Autodesk Fusion 360 part; units mm, degrees
sketch "Sketch1" plane through (0, 0, 0) normal (0, 0, 1) x (1, 0, 0)
  line L0 (44.75, 21) -> (-44.75, 21)
  line L1 (-44.75, 21) -> (-44.75, -21)
  line L2 (-44.75, -21) -> (44.75, -21)
  line L3 (44.75, -21) -> (44.75, 21)
  line L4 (44.75, 21) -> (-44.75, -21) construction
  line L5 (-44.75, 21) -> (44.75, -21) construction
  circle A0 centre (-42.25, 18.5) radius 1.25
  line L6 (20, 0) -> (2.5, 0)
  circle A1 centre (-42.25, -18.5) radius 1.25
  line L7 (0, 2.5) -> (0, 20)
  circle A2 centre (42.25, -18.5) radius 1.25
  circle A3 centre (42.25, 18.5) radius 1.25
  line L8 (38.75, 18.75) -> (-38.75, 18.75)
  line L9 (-38.75, 18.75) -> (-38.75, -18.75)
  line L10 (-38.75, -18.75) -> (38.75, -18.75)
  line L11 (38.75, -18.75) -> (38.75, 18.75)
  line L12 (38.75, 18.75) -> (-38.75, -18.75) construction
  line L13 (-38.75, 18.75) -> (38.75, -18.75) construction
  line L14 (39.75, 19.75) -> (-39.75, 19.75)
  line L15 (-39.75, 19.75) -> (-39.75, -19.75)
  line L16 (-39.75, -19.75) -> (39.75, -19.75)
  line L17 (39.75, -19.75) -> (39.75, 19.75)
  line L18 (39.75, 19.75) -> (-39.75, -19.75) construction
  line L19 (-39.75, 19.75) -> (39.75, -19.75) construction
  line L20 (37.5, 17.5) -> (-37.5, 17.5)
  line L21 (-37.5, 17.5) -> (-37.5, -17.5)
  line L22 (-37.5, -17.5) -> (37.5, -17.5)
  line L23 (37.5, -17.5) -> (37.5, 17.5)
  line L24 (37.5, 17.5) -> (-37.5, -17.5) construction
  line L25 (-37.5, 17.5) -> (37.5, -17.5) construction
  dimension "d5" = 2.5
  dimension "d38" = 75
  dimension "d39" = 35
  dimension "d40" = 3.5
  dimension "d41" = 1.25
  dimension "d42" = 1.25
  dimension "d43" = 1.25
  dimension "d44" = 2.25
  dimension "d45" = 2.5
  dimension "d46" = 2.5
  dimension "d47" = 2.5
extrude "Extrude1" add sketch "Sketch1" along normal blind 2.5 contours L0 L1 L2 L3 | L8 L9 L10 L11 | L14 L15 L16 L17 | L20 L21 L22 L23
extrude "Extrude7" add sketch "Sketch1" along normal blind 5 from surface at 2.5 contours L14 L15 L16 L17
extrude "Extrude8" cut sketch "Sketch1" against normal blind 0.5 from surface at 2.5 contours L20 L21 L22 L23
fillet "Fillet3" radius 2 16 edges at (-39.75, -19.75, 5) (-44.75, -21, 1.25) (-38.75, -18.75, 5) (-37.5, -17.5, 2.25) (-37.5, 17.5, 2.25) (-38.75, 18.75, 5) (-39.75, 19.75, 5) (-44.75, 21, 1.25) (39.75, 19.75, 5) (44.75, 21, 1.25) (39.75, -19.75, 5) (44.75, -21, 1.25) (37.5, -17.5, 2.25) (38.75, -18.75, 5) (38.75, 18.75, 5) (37.5, 17.5, 2.25)
equation "d42 = d41"
equation "d43 = d41"
equation "d44 = d40 - d41"
equation "d45 = d41 + 0.5 * d5"
equation "d46 = d41 + 0.5 * d5"
equation "d47 = d41 + 0.5 * d5"
equation "d48 = d3"
equation "d51 = d3"
Could you check a few things on this model? Use its own coordinates, in mm. A direction names the side the tool comes from. Give positions to 0.01 mm unless a question says otherwise; leave off trailing zeros. Order: outer loops, then holes, each group sorted by start corner. A loop starts at its lowest first (then second) coordinate and runs counter-clockwise, first axis right, second up. Notation, with made-up numbers: (59, 69) - (99, 69) arc R23 cw to (99, 82) - close; hole circle Ø10 at (51.25, 28). An arc over 180 degrees is marked (long way). One line per item, written item: value. Start each with the question number.
1. Imagine slicing it at C-C on y = -13. List the corners of the cut face in (x, z) for me, plus the area to 3 significant figures.
2. Imagine slicing it at B-B on x = -33.5. List the corners of the cut face in (y, z) for me, plus the area to 3 significant figures.
3. Thinking about a two-plate mould opening in X: for faces 1 (the face through (-44.15, 20.43, 1.27)), 2 (the face through (44.18, 20.4, 1.27)), 3 (the face through (-43.24, -17.74, 1.23)), 4 (the face through (0, 19, 7.5)), which applies, +X half, -X half, draft (parallel to the pull), parting line (faces both ways), or undercut?
4. Imagine slicing it at A-A on z = 4.25. List the corners of the cut face in (x, y) for me.
5. If I drill on probe 1 along Y at (x, z) = (-42.25, 1.8); probe 2 along Y at (x, z) = (15, 4); probe 3 along X at (y, z) = (13.5, 3), over which ranges is the centre line in solid material (lowest first)?
6. For P1, Ø1.5, axis at x = -2, z = 5, coming from the -Y side; P2, Ø3, axis at x = -35, y = -14.5, coming from the +Z side; P3, Ø1.5, axis at x = -17, z = 6, coming from the +Y side, each with a flat end and sliding along its axis, tell me the tip position at first contact or that it passes through.
7. For faces 5 (the face through (-39.18, -19.15, 5.04)), 6 (the face through (-1, -19.75, 5)), 7 (the face through (39.75, 0, 5)), 8 (the face through (39.18, 19.15, 5.04)), 9 (the face through (-38.15, 18.18, 5.04)), which set-ups out of +Z, -Z, +X, -X, +Y, -Y let a thin tool reach every point of the face, with its end or its side?
Values:
1. outline: (-44.75, 0) - (44.75, 0) - (44.75, 2.5) - (39.75, 2.5) - (39.75, 7.5) - (38.75, 7.5) - (38.75, 2.5) - (37.5, 2.5) - (37.5, 2) - (-37.5, 2) - (-37.5, 2.5) - (-38.75, 2.5) - (-38.75, 7.5) - (-39.75, 7.5) - (-39.75, 2.5) - (-44.75, 2.5) - close
1. area: 196 mm²
2. outline: (-21, 0) - (21, 0) - (21, 2.5) - (19.75, 2.5) - (19.75, 7.5) - (18.75, 7.5) - (18.75, 2.5) - (17.5, 2.5) - (17.5, 2) - (-17.5, 2) - (-17.5, 2.5) - (-18.75, 2.5) - (-18.75, 7.5) - (-19.75, 7.5) - (-19.75, 2.5) - (-21, 2.5) - close
2. area: 97.5 mm²
3. face 1: -X half
3. face 2: +X half
3. face 3: undercut
3. face 4: draft
4. outline: (-39.75, -17.75) arc R2 ccw to (-37.75, -19.75) - (37.75, -19.75) arc R2 ccw to (39.75, -17.75) - (39.75, 17.75) arc R2 ccw to (37.75, 19.75) - (-37.75, 19.75) arc R2 ccw to (-39.75, 17.75) - close; hole (-38.75, -16.75) arc R2 ccw to (-36.75, -18.75) - (36.75, -18.75) arc R2 ccw to (38.75, -16.75) - (38.75, 16.75) arc R2 ccw to (36.75, 18.75) - (-36.75, 18.75) arc R2 ccw to (-38.75, 16.75) - close
5. probe 1: -21 to -19.75, -17.25 to 17.25, 19.75 to 21
5. probe 2: -19.75 to -18.75, 18.75 to 19.75
5. probe 3: -39.75 to -38.75, 38.75 to 39.75
6. P1: y = -19.75
6. P2: z = 2
6. P3: y = 19.75
7. face 5: +Z, -X, -Y
7. face 6: +Z, +X, -X, -Y
7. face 7: +Z, +X, +Y, -Y
7. face 8: +Z, +X, +Y
7. face 9: +Z
